```python
from build123d import *

# Parameters (mm, degrees)
CUT_EXTRUDE_2_DEPTH            = 70.634269506
HOLE_WIZARD_M1_6_1_D           = 6
HOLE_WIZARD_M1_6_1_CBORE_D     = 12
HOLE_WIZARD_M1_6_1_CBORE_DEPTH = 6
PATTERN_CIRCULAR_1_COUNT       = 5
SKETCH_7_R                     = 9.5
CUT_EXTRUDE_3_DEPTH            = 70.482844453
CUT_EXTRUDE_4_DEPTH            = 70.482844453
PATTERN_CIRCULAR_2_COUNT       = 5
SKETCH_9_R                     = 3
CUT_EXTRUDE_5_DEPTH            = 79.791532331
PATTERN_CIRCULAR_3_COUNT       = 5


with BuildPart() as part:
    # 草图1 → 旋转1 (revolve)
    with BuildSketch(Plane(origin=(0, 0, 0), x_dir=(1, 0, 0), z_dir=(0, 1, 0)), mode=Mode.PRIVATE) as revolve_1_sk:
        with BuildLine():
            Line((0, 0), (-45, 0))
            Line((-45, 0), (-45, 12))
            Line((-45, 12), (-45, 33))
            ThreePointArc((-45, 33), (-42.983093835, 38.686059159), (-36.962809534, 38.291906688))
            Line((-36.962809534, 38.291906688), (-32, 34))
            Line((-32, 34), (-32, 12))
            Line((-32, 12), (0, 12))
            Line((0, 12), (0, 0))
        make_face()
    revolve(revolve_1_sk.sketch.rotate(Axis((0, 0, 0), (0, 0, -1)), 180), axis=Axis((0, 0, 0), (0, 0, -1)))

    # 草图2 → 切除-拉伸2 (cut, through all)
    with BuildSketch(Plane(origin=(0, 0, -12), x_dir=(-1, 0, 0), z_dir=(0, 0, -1))):
        with BuildLine():
            Line((-6, 44.833757456), (-6, 12.649110641))
            ThreePointArc((-6, 12.649110641), (-8.228993532, 11.326237921), (-10.175917134, 9.615129249))
            Line((-10.175917134, 9.615129249), (-40.785335212, 19.560732073))
            ThreePointArc((-40.785335212, 19.560732073), (-26.587560075, 36.594636996), (-6, 44.833757456))
        make_face()
        with BuildLine():
            Line((6, 44.833757456), (6, 12.649110641))
            ThreePointArc((6, 12.649110641), (8.228993532, 11.326237921), (10.175917134, 9.615129249))
            Line((10.175917134, 9.615129249), (40.785335212, 19.560732073))
            ThreePointArc((40.785335212, 19.560732073), (26.587560075, 36.594636996), (6, 44.833757456))
        make_face()
        with BuildLine():
            Line((44.493539145, 8.148053878), (13.884121066, -1.797548946))
            ThreePointArc((13.884121066, -1.797548946), (13.314791228, -4.326237921), (12.289062655, -6.706633958))
            Line((12.289062655, -6.706633958), (31.206723404, -32.74456019))
            ThreePointArc((31.206723404, -32.74456019), (43.019575879, -13.977907527), (44.493539145, 8.148053878))
        make_face()
        with BuildLine():
            Line((21.498519471, -39.797983217), (2.580858723, -13.760056986))
            ThreePointArc((2.580858723, -13.760056986), (0, -14), (-2.580858723, -13.760056986))
            Line((-2.580858723, -13.760056986), (-21.498519471, -39.797983217))
            ThreePointArc((-21.498519471, -39.797983217), (0, -45.23345894), (21.498519471, -39.797983217))
        make_face()
        with BuildLine():
            Line((-31.206723404, -32.74456019), (-12.289062655, -6.706633958))
            ThreePointArc((-12.289062655, -6.706633958), (-13.314791228, -4.326237921), (-13.884121066, -1.797548946))
            Line((-13.884121066, -1.797548946), (-44.493539145, 8.148053878))
            ThreePointArc((-44.493539145, 8.148053878), (-43.019575879, -13.977907527), (-31.206723404, -32.74456019))
        make_face()
    extrude(amount=CUT_EXTRUDE_2_DEPTH, mode=Mode.SUBTRACT)

    # M1.6 六角圆柱头螺钉的柱形沉头孔1 (through all)
    with Locations(Plane(origin=(0, 0, -12), x_dir=(-1, 0, 0), z_dir=(0, 0, -1))):
        with Locations((0, -32)):
            hole_wizard_m1_6_1 = CounterBoreHole(HOLE_WIZARD_M1_6_1_D / 2, HOLE_WIZARD_M1_6_1_CBORE_D / 2, HOLE_WIZARD_M1_6_1_CBORE_DEPTH)

    # 阵列(圆周)1: M1.6 六角圆柱头螺钉的柱形沉头孔1 ×5 about axis
    pattern_circular_1_axis = Axis((0, 0.662193987, 0), (0, 0, 1))
    for i in range(1, PATTERN_CIRCULAR_1_COUNT):
        add(hole_wizard_m1_6_1.rotate(pattern_circular_1_axis, i * 360 / PATTERN_CIRCULAR_1_COUNT), mode=Mode.SUBTRACT)

    # 草图7 → 切除-拉伸3 (cut, through all)
    with BuildSketch(Plane(origin=(0, 0, -12), x_dir=(-1, 0, 0), z_dir=(0, 0, -1))):
        Circle(SKETCH_7_R)
    extrude(amount=-CUT_EXTRUDE_3_DEPTH, mode=Mode.SUBTRACT)

    # 草图7<3> → 切除-拉伸4 (cut, through all)
    with BuildSketch(Plane(origin=(0, 0, -12), x_dir=(-1, 0, 0), z_dir=(0, 0, -1))):
        with BuildLine():
            ThreePointArc((6, 31.432467291), (0, 32), (-6, 31.432467291))
            Line((-6, 31.432467291), (-6, 12.649110641))
            ThreePointArc((-6, 12.649110641), (0, 14), (6, 12.649110641))
            Line((6, 12.649110641), (6, 31.432467291))
        make_face()
    cut_extrude_4 = extrude(amount=-CUT_EXTRUDE_4_DEPTH, mode=Mode.SUBTRACT)

    # 阵列(圆周)2: 切除-拉伸4 ×5 about axis
    pattern_circular_2_axis = Axis((0, 0, 0), (0, 0, 1))
    for i in range(1, PATTERN_CIRCULAR_2_COUNT):
        add(cut_extrude_4.rotate(pattern_circular_2_axis, i * 360 / PATTERN_CIRCULAR_2_COUNT), mode=Mode.SUBTRACT)

    # 草图9 → 切除-拉伸5 (cut, through all)
    with BuildSketch(Plane(origin=(6, 0, 0), x_dir=(0, 0, -1), z_dir=(1, 0, 0))):
        with Locations(Location((33, 38, 0), (0, 0, 90))):
            Circle(SKETCH_9_R)
        with Locations(Location((20, 38, 0), (0, 0, 90))):
            Circle(SKETCH_9_R)
    cut_extrude_5 = extrude(amount=-CUT_EXTRUDE_5_DEPTH, mode=Mode.SUBTRACT)

    # 阵列(圆周)3: 切除-拉伸5 ×5 about axis
    pattern_circular_3_axis = Axis((0, 0, 0), (0, 0, -1))
    for i in range(1, PATTERN_CIRCULAR_3_COUNT):
        add(cut_extrude_5.rotate(pattern_circular_3_axis, i * 360 / PATTERN_CIRCULAR_3_COUNT), mode=Mode.SUBTRACT)


solid = part.part
```
Build history of the part. All positions in model axes, mm. A direction names the side the tool comes from. Coordinates: 2 decimals unless noted, no trailing zeros. Order: outer loops, then holes, each group sorted by start corner. A loop starts at its lowest first (then second) coordinate and runs counter-clockwise, first axis right, second up. Notation, with made-up numbers: (23, 1) -> (47, 1) arc R27 ccw to (47, 19) -> close; hole circle Ø3 at (-0.75, -30.5). An arc over 180 degrees is marked (long way). Answer in a Markdown table with one row per item. Add a question column.
Q1. Band-saw the part on A-A, the plane x = 0. List the corners of the cut face in (y, z), then the cut area to 3 significant figures.
Q2. Drop flat-ended pins along their axis: pin 1 (6 mm diameter, centred on x = 16, y = 25, fed in from -Z); pin 2 (8 mm diameter, centred on x = 33, z = -4, fed in from -Y); pin 3 (9.5 mm diameter, centred on x = 31.06, y = -9.43, fed in from -Z). Give the stop position or say it passes through.
Q3. Which spindle directions (+Z, -Z, +X, -X, +Y, -Y) get a long thin tool onto all of the face, cutting with end or side? Do faces 1 (the face through (18, 30, -6)), 2 (the face through (20.321, -27.814, -36.116)), 3 (the face through (17.505, -34.301, -25.566)). Say none if no direction does.
Q4. Wall check: line 1 along Y through (x, z) = (0, -9.65); line 2 along Y through (x, z) = (0, -2); line 3 along Z through (x, y) = (2, 38). Give the ranges that are in metal, low to high. Write a range as [from, to].
Q5. Mould opens along X. For faces 4 (the face through (6, 38, -26)), 5 (the face through (13.341, 4.244, -6.084)), 6 (the face through (-8.024, -21.252, -6.084)), 7 (the face through (-27.213, -27.248, -25.566)) say: +X half, -X half, draft (parallel to the pull), parting line (faces both ways), or undercut.
Q6. Band-saw the part on B-B, the plane y = -8. Give the number of separate pieces and of enclosed holes in the cut face, then the cut area to 3 significant figures.
Answers follow:
| question | item | result |
|---|---|---|
| 1 | outline | (-45, -12) -> (-38, -12) -> (-38, -6) -> (-35, -6) -> (-35, 0) -> (-45, 0) -> close; (-29, -6) -> (-26, -6) -> (-26, -12) -> (-9.5, -12) -> (-9.5, 0) -> (-29, 0) -> close; (9.5, -12) -> (14, -12) -> (14, 0) -> (9.5, 0) -> close; (32, -34) -> (36.96, -38.29) arc R5 ccw to (45, -33) -> (45, 0) -> (32, 0) -> close; hole circle Ø6 at (38, -33); hole circle Ø6 at (38, -20) |
| 1 | area | 807 mm^2 |
| 2 | pin 1 | z = -12 |
| 2 | pin 2 | y = -34.41 |
| 2 | pin 3 | z = -6 |
| 3 | face 1 | -Z |
| 3 | face 2 | -Z, +Y |
| 3 | face 3 | -Z, -Y |
| 4 | line 1 | [-45, -38], [-26, -9.5], [9.5, 14], [32, 45] |
| 4 | line 2 | [-45, -35], [-29, -9.5], [9.5, 14], [32, 45] |
| 4 | line 3 | [-39.01, -36], [-30, -23], [-17, 0] |
| 5 | face 4 | +X half |
| 5 | face 5 | undercut |
| 5 | face 6 | undercut |
| 5 | face 7 | -X half |
| 6 | separate pieces | 6 |
| 6 | enclosed holes | 0 |
| 6 | area | 695 mm^2 |
